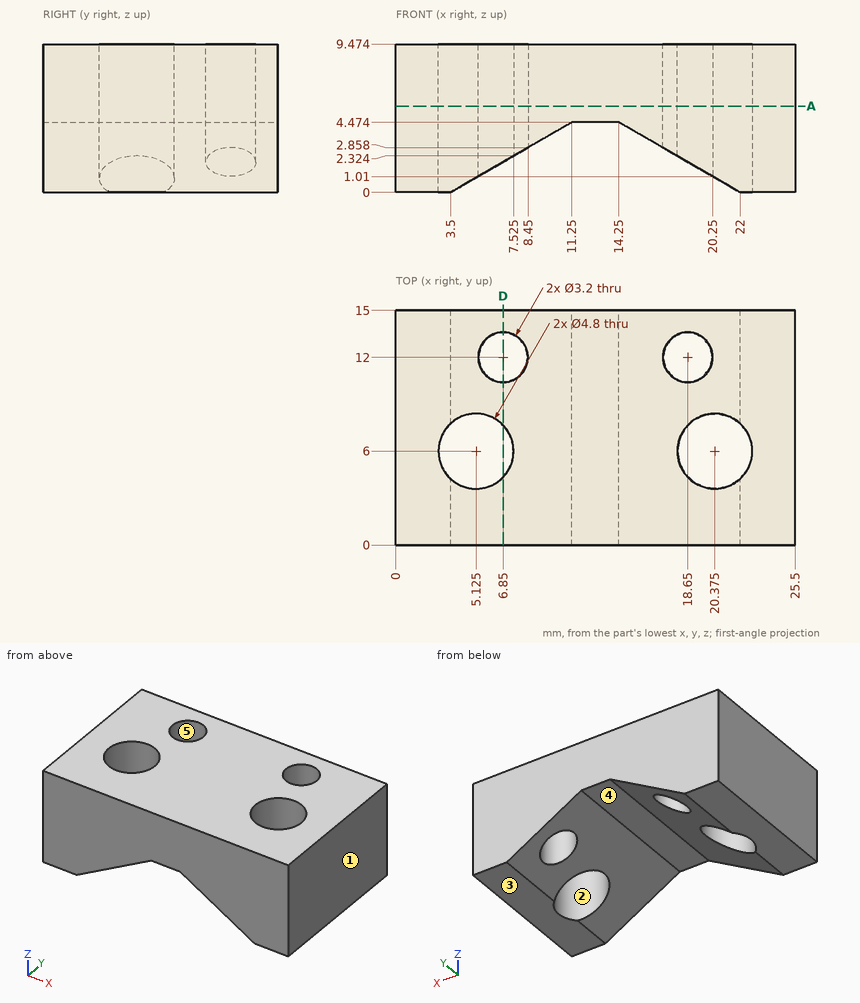
For this review, use the dimensioned drawing (mm, ordinates from the lowest corner) and the shaded views. A direction names the side the tool comes from. Give positions to 0.01 mm unless a question says otherwise; leave off trailing zeros. Order: outer loops, then holes, each group sorted by start corner. A loop starts at its lowest first (then second) coordinate and runs counter-clockwise, first axis right, second up. Notation, with made-up numbers: (52.25, 36) - (57.25, 36) arc R25 cw to (57.25, 55) - close; hole circle Ø3 at (-1, 4.5). An arc over 180 degrees is marked (long way). Use CSV: the item, a comma, the result in double quotes. Start each with the question number.
Q1. Machinability: for the marked faces 4 and 5, which of the approach directions +Z, -Z, +X, -X, +Y, -Y give a long, thin tool a straight path to every point of the face, cutting with its end or side? Answer none if there is none.
Q2. Draft analysis for pull direction X (two halves, no side actions). For the marked faces 1, 2 and 3, state which applies: pulls with the +X half, pulls with the -X half, needs draft (parallel to the pull), parting line crosses it, or undercut.
Q3. For P1, Ø4, axis at x = 18.65, y = 12, coming from the -Z side; P2, Ø5, axis at x = 19, y = 12, coming from the -Z side; P3, Ø0.9, axis at x = 12, y = 7.5, coming from the -Z side, all flat-tipped, find the tip position at first contact; note any pin that passes through.
Q4. For line 1 (X direction, y = 12, z = 5.25); line 2 (X direction, y = 6, z = 7.75) (1 decimal); line 3 (Y direction, x = 18.65, z = 7.5), list the stretches that pass through material, from the lowest coordinate up.
Q5. Take a section at A-A (z = 5.5). Count the separate pieces of the cut face and the enclosed holes in it, and give its area (3 significant figures).
Q6. Take a section at D-D (x = 6.85). State the section outline as (y, z) points (1 decimal).
Calculated:
1,face 4,"-Z, +Y, -Y"
1,face 5,"+Z, -Z"
2,face 1,"pulls with the +X half"
2,face 2,"undercut"
2,face 3,"needs draft"
3,P1,"stops at z = 0.78"
3,P2,"stops at z = 0.29"
3,P3,"stops at z = 4.47"
4,line 1,"x = 0 to 5.25, 8.45 to 17.05, 20.25 to 25.5"
4,line 2,"x = 0 to 2.7, 7.5 to 18, 22.8 to 25.5"
4,line 3,"y = 0 to 4.33, 7.67 to 10.4, 13.6 to 15"
5,separate pieces,"1"
5,enclosed holes,"4"
5,area,"330 mm²"
6,outline,"(0, 1.9) - (4.3, 1.9) - (4.3, 9.5) - (0, 9.5) - close; (7.7, 1.9) - (10.4, 1.9) - (10.4, 9.5) - (7.7, 9.5) - close; (13.6, 1.9) - (15, 1.9) - (15, 9.5) - (13.6, 9.5) - close"
